Can you work these out from the model? Positions are in its coordinate system, mm. A direction names the side the tool comes from. Round coordinates to 2 decimals unless told otherwise and drop trailing zeros. Order: outer loops, then holes, each group sorted by start corner. A loop starts at its lowest first (then second) coordinate and runs counter-clockwise, first axis right, second up. Notation, with made-up numbers: (52.25, 0) -> (80.25, 0) arc R27 cw to (80.25, 29) -> close; hole circle Ø5 at (-16.75, 42). An arc over 180 degrees is marked (long way). One line per item, written item: value.
Autodesk Fusion 360 part; units mm, degrees
sketch "Sketch1" plane through (0, 0, 0) normal (0, 0, 1) x (1, 0, 0) in component "Jackson's Editing ATK"
  line L0 (-33.4351, 34.2031) -> (6.9349, 34.2031)
  line L1 (6.9349, 34.2031) -> (6.9349, 96.1631)
  line L2 (6.9349, 96.1631) -> (-33.4351, 96.1631)
  line L3 (-33.4351, 96.1631) -> (-33.4351, 34.2031)
  line L4 (-42.9351, 105.6631) -> (17.4349, 105.6631)
  line L5 (17.4349, 105.6631) -> (17.4349, 23.7031)
  line L6 (17.4349, 23.7031) -> (-42.9351, 23.7031)
  line L7 (-42.9351, 23.7031) -> (-42.9351, 105.6631)
  circle A0 centre (-37.9351, 28.7031) radius 1.7
  circle A1 centre (-37.9351, 28.7031) radius 3
  circle A2 centre (12.4349, 28.7031) radius 1.7
  circle A3 centre (12.4349, 28.7031) radius 1.7
  circle A4 centre (12.4349, 28.7031) radius 3
  circle A5 centre (12.4349, 100.6631) radius 1.7
  circle A6 centre (12.4349, 100.6631) radius 3
  circle A7 centre (-37.9351, 100.6631) radius 1.7
  circle A8 centre (-37.9351, 100.6631) radius 3
  dimension "d1" = 61.96
  dimension "d2" = 40.37
  dimension "d3" = 60.37
  dimension "d4" = 81.96
  dimension "d5" = 9.5
  dimension "d6" = 9.5
  dimension "d7" = 3.4
  dimension "d8" = 5
  dimension "d9" = 5
  dimension "d17" = 6
  dimension "d20" = 3.4
  dimension "d21" = 5
  dimension "d22" = 5
  dimension "d23" = 3.4
  dimension "d24" = 6
  dimension "d25" = 3.4
  dimension "d26" = 5
  dimension "d27" = 5
  dimension "d28" = 6
  dimension "d29" = 3.4
  dimension "d30" = 5
  dimension "d31" = 5
  dimension "d32" = 6
extrude "Extrude1" add sketch "Sketch1" along normal blind 9.9 from surface at 3.1 contours A1 | A4 | A6 | A8 makes body 1 at (-34.9388, 28.5536, 9.7) makes body 2 at (-35.3752, 102.2274, 9.7) makes body 3 at (15.4312, 28.5536, 9.7) makes body 4 at (15.254, 99.6371, 9.7) in component "Jackson's Editing ATK"
extrude "Extrude2" add sketch "Sketch1" along normal blind 13 contours L4 L5 L6 L7 bodies 1 2 3 4 in component "Jackson's Editing ATK"
extrude "Extrude3" add sketch "Sketch1" along normal blind 3 contours L0 L1 L2 L3 bodies 1 in component "Jackson's Editing ATK"
sketch "Sketch2" plane through (0, 0, 13) normal (0, 0, 1) x (-1, 0, 0) in component "Jackson's Editing ATK"
  circle A0 centre (37.9351, -28.7031) radius 1.7
  circle A1 centre (-12.4349, -100.6631) radius 1.7
  line L0 (33.4351, -34.2031) -> (33.4351, -96.1631)
  line L1 (33.4351, -96.1631) -> (-6.9349, -96.1631)
  line L2 (-6.9349, -96.1631) -> (-6.9349, -34.2031)
  line L3 (-6.9349, -34.2031) -> (33.4351, -34.2031)
  line L4 (42.9351, -23.7031) -> (-17.4349, -23.7031)
  line L5 (-17.4349, -23.7031) -> (-17.4349, -105.6631)
  line L6 (-17.4349, -105.6631) -> (42.9351, -105.6631)
  line L7 (42.9351, -105.6631) -> (42.9351, -23.7031)
  circle A2 centre (37.9351, -100.6631) radius 1.7
  circle A3 centre (-12.4349, -28.7031) radius 1.7
  line L8 (21.4871, -96.1631) -> (2.9871, -96.1631)
  line L9 (2.9871, -96.1631) -> (2.9871, -105.6631)
  line L10 (2.9871, -105.6631) -> (21.4871, -105.6631)
  line L11 (21.4871, -105.6631) -> (21.4871, -96.1631)
  dimension "d40" = 21.448
  dimension "d41" = 18.5
extrude "Extrude4" cut sketch "Sketch2" against normal blind 7.5 contours L1 L6 L8 L9 L10 L11 bodies 1 in component "Jackson's Editing ATK"
fillet "Fillet1" radius 5.5 1 edges at (-42.9351, 23.7031, 6.5) on bodies 1 in component "Jackson's Editing ATK"
fillet "Fillet2" radius 5.5 1 edges at (17.4349, 23.7031, 6.5) on bodies 1 in component "Jackson's Editing ATK"
fillet "Fillet3" radius 5.5 1 edges at (17.4349, 105.6631, 6.5) on bodies 1 in component "Jackson's Editing ATK"
fillet "Fillet4" radius 5.5 1 edges at (-42.9351, 105.6631, 6.5) on bodies 1 in component "Jackson's Editing ATK"
component "Jackson's Editing ATK" placed x (1, 0, 0) y (0, 1, 0) z (0, 0, 1) at (0, 0, 0)
Q1. Please list where these lines run through material, in increasing order: line 1 along Y through (x, z) = (-28, 12); line 2 along X through (y, z) = (102, 8.5) (3 decimals); line 3 along X through (y, z) = (56, 6.5).
Answers below:
line 1: 23.7 to 34.2, 96.16 to 105.66
line 2: -42.619 to -38.985, -36.885 to -21.487, -2.987 to 11.385, 13.485 to 17.119
line 3: -42.94 to -33.44, 6.93 to 17.43
Q2. I want a section at C-C on z = 1. List the corners of the cut face in (x, y) for me, plus the area to 3 significant figures.
Answers below:
outline: (-42.94, 29.2) arc R5.5 ccw to (-37.44, 23.7) -> (11.93, 23.7) arc R5.5 ccw to (17.43, 29.2) -> (17.43, 100.16) arc R5.5 ccw to (11.93, 105.66) -> (-37.44, 105.66) arc R5.5 ccw to (-42.94, 100.16) -> close; hole circle Ø6 at (-37.94, 28.7); hole circle Ø6 at (-37.94, 100.66); hole circle Ø6 at (12.43, 28.7); hole circle Ø6 at (12.43, 100.66)
area: 4,810 mm^2
Q3. I want a section at D-D on z = 9.25. List the corners of the cut face in (x, y) for me.
Answers below:
outline: (-42.94, 29.2) arc R5.5 ccw to (-37.44, 23.7) -> (11.93, 23.7) arc R5.5 ccw to (17.43, 29.2) -> (17.43, 100.16) arc R5.5 ccw to (11.93, 105.66) -> (-2.99, 105.66) -> (-2.99, 96.16) -> (6.93, 96.16) -> (6.93, 34.2) -> (-33.44, 34.2) -> (-33.44, 96.16) -> (-21.49, 96.16) -> (-21.49, 105.66) -> (-37.44, 105.66) arc R5.5 ccw to (-42.94, 100.16) -> close; hole circle Ø3.4 at (-37.94, 28.7); hole circle Ø3.4 at (-37.94, 100.66); hole circle Ø3.4 at (12.43, 28.7); hole circle Ø3.4 at (12.43, 100.66)
Q4. I want a section at B-B on x = -23.5. List the corners of the cut face in (y, z) for me, plus the area to 3 significant figures.
Answers below:
outline: (23.7, 0) -> (105.66, 0) -> (105.66, 13) -> (96.16, 13) -> (96.16, 3) -> (34.2, 3) -> (34.2, 13) -> (23.7, 13) -> close
area: 446 mm^2
Q5. On a 3-axis mill with a long thin cutter (end or side, diameter ignored), from which of +Z, -Z, +X, -X, +Y, -Y can I reach the whole of each face in a straight line? I mean faces 5 (the face through (-12, 101, 5.5)), 6 (the face through (-14, 66, 3)), 7 (the face through (14, 27, 3.1)). Say none if no direction works.
Answers below:
face 5: +Z, +Y
face 6: +Z
face 7: -Z
Q6. We'd pull the mould along Y, two halves only. Please class faces 1 (the face through (-41.281, 104.095, 6.591)), 2 (the face through (-12, 23.703, 6)), 3 (the face through (-2.987, 101, 9)), 4 (the face through (6.935, 65, 8)): released by +Y, released by -Y, zero draft, split by the parting line, or undercut.
Answers below:
face 1: released by +Y
face 2: released by -Y
face 3: zero draft
face 4: undercut
Q7. Will these pins go through, and if not, where does the flat tip stop? pin 1 Ø7.5 at (x, y) = (-7.5, 101) entering from +Z; pin 2 Ø3 at (x, y) = (-39, 100) entering from -Z; pin 3 Ø12 at (x, y) = (-10, 55.5) entering from +Z.
Answers below:
pin 1: z = 5.5
pin 2: z = 3.1
pin 3: z = 3
Q8. I want a section at A-A on y = 43. List the corners of the cut face in (x, z) for me.
Answers below:
outline: (-42.94, 0) -> (17.43, 0) -> (17.43, 13) -> (6.93, 13) -> (6.93, 3) -> (-33.44, 3) -> (-33.44, 13) -> (-42.94, 13) -> close
